Verification items for the finished model (mm, model axes). A direction names the side the tool comes from. Round coordinates to 2 decimals unless told otherwise and drop trailing zeros. Write each loop counter-clockwise with the first axis right and the second up, starting at its lowest first coordinate (ties: lowest second). Pieces come first, ordered by that corner, then holes.
Autodesk Inventor part; units mm, degrees
ref_plane "YZ Plane" through (0, 0, 0) normal (1, 0, 0) x (0, 1, 0)
ref_plane "XZ Plane" through (0, 0, 0) normal (0, 1, 0) x (-1, 0, 0)
ref_plane "XY Plane" through (0, 0, 0) normal (0, 0, 1) x (1, 0, 0)
sketch "Szkic7" plane through (0, 0, 0) normal (0, 0, 1) x (1, 0, 0)
  circle A0 centre (0, 0) radius 16.6245
  dimension "d35" = 33.249
extrude "Wyciągnięcie proste2" add sketch "Szkic7" along normal mid plane 21.3875
chamfer "Faza2" distance 1 angle 45 1 edges at (-16.6245, 0, 10.6938)
sketch "Szkic9" plane through (0, 0, 10.6938) normal (0, 0, 1) x (1, 0, 0)
  circle A0 centre (0, 0) radius 15.6245
extrude "Wyciągnięcie proste3" add sketch "Szkic9" along normal blind 1.8125
sketch "Szkic10" plane through (0, 0, 12.5063) normal (0, 0, 1) x (1, 0, 0)
  line L0 (-10.3923, 18) -> (10.3923, 18)
  line L1 (10.3923, 18) -> (20.7846, 0)
  line L2 (20.7846, 0) -> (10.3923, -18)
  line L3 (10.3923, -18) -> (-10.3923, -18)
  line L4 (-10.3923, -18) -> (-20.7846, 0)
  line L5 (-20.7846, 0) -> (-10.3923, 18)
  line L6 (0, 23.2743) -> (0, -23.2743) construction
  line L7 (-23.2743, 0) -> (23.2743, 0) construction
  point P0 (0, 0)
  point P1 (0, 0)
  point P2 (0, 18)
  dimension "d44" = 36
extrude "Wyciągnięcie proste4" add sketch "Szkic10" along normal blind 5.8
sketch "Szkic12" plane through (0, 0, 0) normal (0, 1, 0) x (-1, 0, 0)
  line L0 (0, -2.1463) -> (0, 12.8775) construction
  line L1 (-10.3923, 12.5063) -> (-10.3923, 18.3063) construction
  line L2 (-20.7846, 18.3063) -> (-10.3923, 18.3063) construction
  line L3 (-20.7846, 12.5063) -> (-20.7846, 18.3063)
  line L4 (-20.7846, 17.6632) -> (-18.3846, 18.3063)
  line L5 (-20.7846, 18.3063) -> (-10.3923, 18.3063)
  line L6 (-20.7846, 12.5063) -> (-10.3923, 12.5063)
  point P0 (0, 0)
  dimension "d50" = 15
  dimension "d51" = 2.4
revolve "Obrót2" cut sketch "Szkic12" angle 360 about axis through (0, 0, -10) along (0, 0, 1)
thread "Gwint3"
chamfer "Faza3" distance 1 angle 45 1 edges at (-16.6245, 0, -10.6938)
equation "\"d35\" = OD"
equation "\"d36\" = 0.7375 * L"
equation "\"d42\" = 0.0625 * L"
equation "\"d44\" = SW"
equation "\"d45\" = 0.2 * L"
equation "\"d51\" = 0.0666667 * SW"
equation "\"SzerokośćGięciaPodcięcia\" = Grubość"
equation "\"RozmiarPodcięciaNarożnika\" = 4 * Grubość"
equation "\"PromieńPrzejścia\" = PromieńGięcia"
equation "\"Rozmiar_promienia_Jacobiego\" = PromieńGięcia"
equation "\"Wielk_odstępu\" = Grubość"
equation "\"d2\" = PromieńGięcia"
equation "\"d23\" = PromieńGięcia"
equation "\"OD\" = 33.249"
equation "\"SW\" = 36"
equation "\"L\" = 29"
properties part number "Korek sześciokątny BSP 1'' L=29" material "304"
Q1. Sectioned sample at A-A (x = 0). Enter the section's corners in (y, z).
Recorded:
outline: (-18, 12.51) - (-15.62, 12.51) - (-15.62, 10.69) - (-16.62, 9.69) - (-16.62, -9.69) - (-15.62, -10.69) - (15.62, -10.69) - (16.62, -9.69) - (16.62, 9.69) - (15.62, 10.69) - (15.62, 12.51) - (18, 12.51) - (18, 18.31) - (-18, 18.31) - close
Q2. Depth check by flat-ended pin: P1, Ø1, axis at y = -5.5, z = -5.5, coming from the -X side; P2, Ø1.5, axis at x = 15.5, z = 14.5, coming from the -Y side; P3, Ø3, axis at y = 7.5, z = 8.5, coming from the -X side. Enter the tip coordinate at first touch or a pass-through.
Recorded:
P1: stops at x = -15.85
P2: stops at y = -10.45
P3: stops at x = -15.5
Q3. Release check for a two-part mould opening along Z. For faces 1 (the conical face through (-9.46, -16.556, 18.123)), 2 (the flat face through (15.3, 4.1, 12.506)), 3 (the cylindrical face through (14.9, -4.7, 11.6)), 4 (the flat face through (0, 18, 15)) record: released by +Z, released by -Z, zero draft, split by the parting line, or undercut.
Recorded:
face 1: released by +Z
face 2: undercut
face 3: undercut
face 4: zero draft
Q4. Material ranges on line 1 along Z through (x, y) = (-8, 14); line 2 along Z through (x, y) = (-7.5, -15.5); line 3 along X through (y, z) = (5, -8), recorded low to high.
Recorded:
line 1: z = -10.19 to 10.19, 12.51 to 18.31
line 2: z = 12.51 to 18.31
line 3: x = -15.85 to 15.85
Q5. Tool access check on faces 5 (the flat face through (-15.661, 8.874, 15.366)), 6 (the cylindrical face through (-3.6, 16.23, -0.14)). Record the directions out of +Z, -Z, +X, -X, +Y, -Y that give a thin tool (end or side, any length) a straight path to the whole face; none if there is none.
Recorded:
face 5: +Z, -Z, -X, +Y
face 6: -Z
Q6. Sectioned sample at B-B (z = 16.5). Enter the section's corners in (x, y), plus the area to 3 significant figures.
Recorded:
outline: (-20.78, 0) - (-10.39, -18) - (10.39, -18) - (20.78, 0) - (10.39, 18) - (-10.39, 18) - close
area: 1,120 mm2
Q7. Sectioned sample at C-C (z = -0.75). Enter the section's corners in (x, y), plus the area to 3 significant figures.
Recorded:
outline: circle Ø33.25 at (0, 0)
area: 868 mm2
